CAD build for the part. Positions are in the model's coordinates, mm. A direction names the side the tool comes from. Give positions to 0.01 mm unless a question says otherwise; leave off trailing zeros. Loops run counter-clockwise (first coordinate to the right, second up) from the corner with the lowest first, then second, coordinate; pieces in that order, holes last. Notation, with made-up numbers: (-5.75, -5.5) - (34.25, -5.5) arc R34 cw to (34.25, 29.5) - close; hole circle Ø7 at (84.25, 46.25). An arc over 180 degrees is marked (long way). Return JSON: item names as keys, results as strings.
from build123d import *

# Parameters (mm, degrees)
PAD_DEPTH       = 5
POCKET_DEPTH    = 4
SKETCH002_R     = 1.6
POCKET001_DEPTH = 5
FILLET_R        = 2
CHAMFER_SIZE    = 0.5


with BuildPart() as part:
    # Sketch → Pad (new body, symmetric)
    with BuildSketch(Plane.XZ):
        Polygon((-22.5, 0), (-20, 5), (20, 5), (22.5, 0), align=None)
    extrude(amount=PAD_DEPTH, both=True)

    # Sketch001 → Pocket (cut)
    with BuildSketch(Plane(origin=(0, 0, 5), x_dir=(-1, 0, 0), z_dir=(0, 0, 1))):
        Polygon((-14.075, 2.72798), (-10.925, 2.72798), (-9.35, 0), (-10.925, -2.72798), (-14.075, -2.72798), (-15.65, 0), align=None)
        Polygon((10.925, 2.72798), (14.075, 2.72798), (15.65, 0), (14.075, -2.72798), (10.925, -2.72798), (9.35, 0), align=None)
    extrude(amount=-POCKET_DEPTH, mode=Mode.SUBTRACT)

    # Sketch002 → Pocket001 (cut)
    with BuildSketch(Plane(origin=(0, 0, 0), x_dir=(1, 0, 0), z_dir=(0, 0, -1))):
        with Locations((-12.5, 0)):
            Circle(SKETCH002_R)
        with Locations((12.5, 0)):
            Circle(SKETCH002_R)
    extrude(amount=-POCKET001_DEPTH, mode=Mode.SUBTRACT)

    # Fillet
    fillet_edges = [part.edges().sort_by_distance(p)[0] for p in [
        (20, 0, 5),
        (-20, 0, 5),
        (0, -5, 5),
        (0, 5, 5),
    ]]
    fillet(fillet_edges, radius=FILLET_R)

    # Chamfer
    chamfer_edges = [part.edges().sort_by_distance(p)[0] for p in [
        (-14.1, 0, 0),
        (10.9, 0, 0),
        (22.5, 0, 0),
        (0, 5, 0),
        (0, -5, 0),
        (-22.5, 0, 0),
    ]]
    chamfer(chamfer_edges, length=CHAMFER_SIZE)


solid = part.part
1. Drill centre lines: probe 1 along Y at (x, z) = (-12.5, 0.7); probe 2 along X at (y, z) = (0, 0.95) (3 decimals); probe 3 along X at (y, z) = (0, 0.85) (3 decimals). Where is each one in solid material? Low to high.
Values follow:
{"probe 1": "y = -5 to -1.6, 1.6 to 5", "probe 2": "x = -22.025 to -14.1, -10.9 to 10.9, 14.1 to 22.025", "probe 3": "x = -22.075 to -14.1, -10.9 to 10.9, 14.1 to 22.075"}
2. Which spindle directions (+Z, -Z, +X, -X, +Y, -Y) get a long thin tool onto all of the face, cutting with end or side? Do faces 4 (the face through (-21.427, -0.07, 2.147)), 5 (the face through (-14.851, -1.383, 3.028)). Say none if no direction does.
Values follow:
{"face 4": "+Z, -X, +Y, -Y", "face 5": "+Z"}
3. Cut at C-C, the plane y = 0.5. Give the number of separate pieces and of enclosed holes in the cut face, plus the area to 3 significant figures.
Values follow:
{"separate pieces": "3", "enclosed holes": "0", "area": "159 mm²"}
4. Drop flat-ended pins along their axis: P1, Ø1, axis at x = 13.5, y = 2, coming from the +Z side; P2, Ø1.5, axis at y = 1.5, z = 1.5, coming from the +X side (3 decimals); P3, Ø4, axis at x = -12.5, y = 0, coming from the -Z side. Give the stop position or say it passes through.
Values follow:
{"P1": "stops at z = 1", "P2": "stops at x = 22.125", "P3": "stops at z = 0.1"}
5. Cut at A-A, the plane z = 1.6. Write the cut outline in (x, y) (3 decimals).
Values follow:
{"outline": "(-21.7, -5) - (21.7, -5) - (21.7, 5) - (-21.7, 5) - close; hole (-15.65, 0) - (-14.075, -2.728) - (-10.925, -2.728) - (-9.35, 0) - (-10.925, 2.728) - (-14.075, 2.728) - close; hole (9.35, 0) - (10.925, -2.728) - (14.075, -2.728) - (15.65, 0) - (14.075, 2.728) - (10.925, 2.728) - close"}
6. Pull direction X, two halves, no side cores. Call faces 1 (the face through (0, 0, 0)), 2 (the face through (19.8, 0.07, 4.71)), 3 (the face through (12, 2.728, 3)): +X half, -X half, draft (parallel to the pull), parting line (faces both ways), or undercut.
Values follow:
{"face 1": "draft", "face 2": "+X half", "face 3": "undercut"}
7. Cut at B-B, the plane x = -12.5. Write the cut outline in (y, z), plus the area to 3 significant figures.
Values follow:
{"outline": "(-5, 0.5) - (-4.5, 0) - (-2.1, 0) - (-1.6, 0.5) - (-1.6, 1) - (-2.73, 1) - (-2.73, 5) - (-3, 5) arc R2 ccw to (-5, 3) - close; (1.6, 0.5) - (2.1, 0) - (4.5, 0) - (5, 0.5) - (5, 3) arc R2 ccw to (3, 5) - (2.73, 5) - (2.73, 1) - (1.6, 1) - close", "area": "22.8 mm²"}
8. Cut at D-D, the plane x = -5. Write the cut outline in (y, z), plus the area to 3 significant figures.
Values follow:
{"outline": "(-5, 0.5) - (-4.5, 0) - (4.5, 0) - (5, 0.5) - (5, 3) arc R2 ccw to (3, 5) - (-3, 5) arc R2 ccw to (-5, 3) - close", "area": "48.0 mm²"}
